Study the drawing (mm; zero at the part's minimum x, y, z) and answer. A direction names the side the tool comes from. Coordinates: 2 decimals unless noted, no trailing zeros. Order: outer loops, then holes, each group sorted by start corner. A loop starts at its lowest first (then second) coordinate and runs counter-clockwise, first axis right, second up. Notation, with made-up numbers: (2.5, -14) -> (39.5, -14) arc R6 cw to (39.5, -5) -> close; hole circle Ø1 at (9, 20). An arc over 180 degrees is marked (long way). Write each question's results on one line, items separated by ' | '. Start each with the question number.
(1) The part is cut by section B-B, the plane z = 45.5. Give the vertices of the cut face in (x, y), then the cut area to 3 significant figures.
(2) The part is cut by section D-D, the plane x = 92.5. Give the vertices of the cut face in (y, z).
(3) Determine the mould class of the marked faces 3, 4 and 5 for opening direction X: +X half, -X half, draft (parallel to the pull), parting line (faces both ways), or undercut.
(4) The part is cut by section A-A, the plane x = 185. Give the vertices of the cut face in (y, z), then the cut area to 3 significant figures.
(5) A tool of negligible diameter and unlimited length cuts with its end or side. For the marked faces 1 and 2, from which of +Z, -Z, +X, -X, +Y, -Y can it reach the whole face along a straight path? Write none if from no direction.
(6) Straight lines are drawn through the part: L1, parallel to Z at x = 210, y = 11.5; L2, parallel to X at y = 4.25, z = 32; L3, parallel to X at y = 10.75, z = 36.5 (1 decimal). For each, find the intervals that lie inside material, in ascending order.
(7) The part is cut by section C-C, the plane x = 160. Give the vertices of the cut face in (y, z) (1 decimal).
(8) Given pin 1 (5 mm diameter, centred on x = 81, y = 6, fed in from +Z); pin 2 (1 mm diameter, centred on x = 160.5, y = 12, fed in from +Z); pin 3 (4.5 mm diameter, centred on x = 38, y = 8.5, fed in from -Z) (1 decimal), each flat-ended and moving along its own axis, determine where each tip first touches the part or whether it passes through.
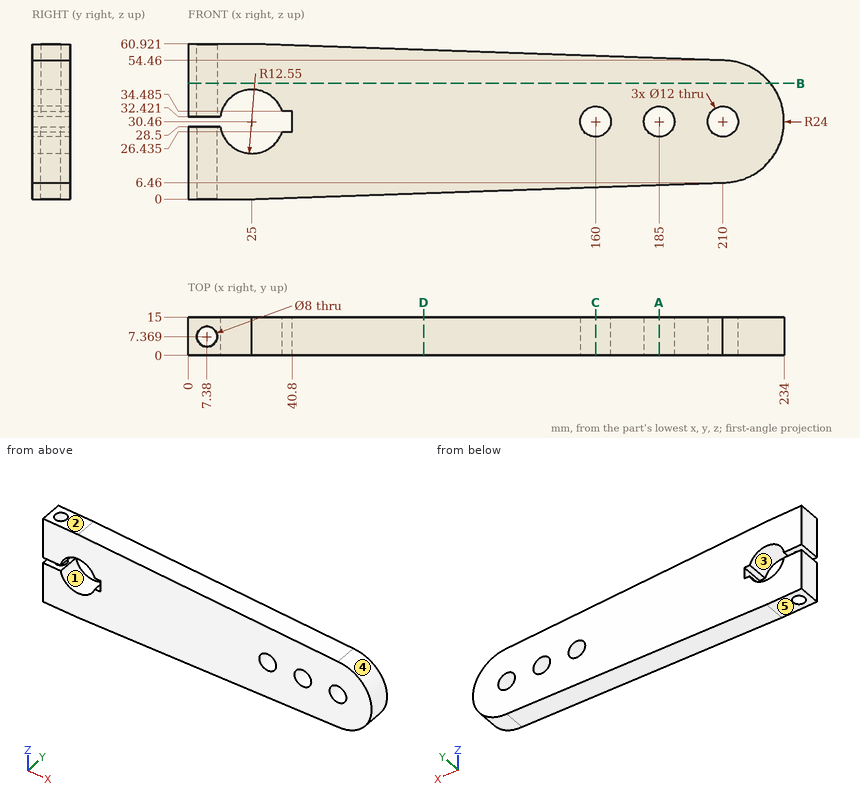
Established:
1) outline: (0, 0) -> (228.7, 0) -> (228.7, 15) -> (0, 15) -> close; hole circle Ø8 at (7.38, 7.37) | area: 3,380 mm^2
2) outline: (0, 2.36) -> (15, 2.36) -> (15, 58.56) -> (0, 58.56) -> close
3) face 3: undercut | face 4: +X half | face 5: draft
4) outline: (0, 5.59) -> (15, 5.59) -> (15, 24.46) -> (0, 24.46) -> close; (0, 36.46) -> (15, 36.46) -> (15, 55.33) -> (0, 55.33) -> close | area: 566 mm^2
5) face 1: +Y, -Y | face 2: +Z, +X, -X, +Y, -Y
6) L1: z = 6.46 to 24.46, 36.46 to 54.46 | L2: x = 40.8 to 154.2, 165.8 to 179.2, 190.8 to 204.2, 215.8 to 233.95 | L3: x = 0 to 5.2, 9.5 to 14, 36 to 233.2
7) outline: (0, 4.7) -> (15, 4.7) -> (15, 24.5) -> (0, 24.5) -> close; (0, 36.5) -> (15, 36.5) -> (15, 56.2) -> (0, 56.2) -> close
8) pin 1: stops at z = 59.05 | pin 2: stops at z = 56.21 | pin 3: stops at z = 0.4
